The model under review builds one solid part; all positions refer to its coordinate system, in mm. Face numbers are marked on the shaded views. A direction names the side the tool comes from. Give positions to 0.01 mm unless a question says otherwise; leave off trailing zeros. Order: outer loops, then holes, each group sorted by start corner. A loop starts at its lowest first (then second) coordinate and runs counter-clockwise, first axis right, second up.
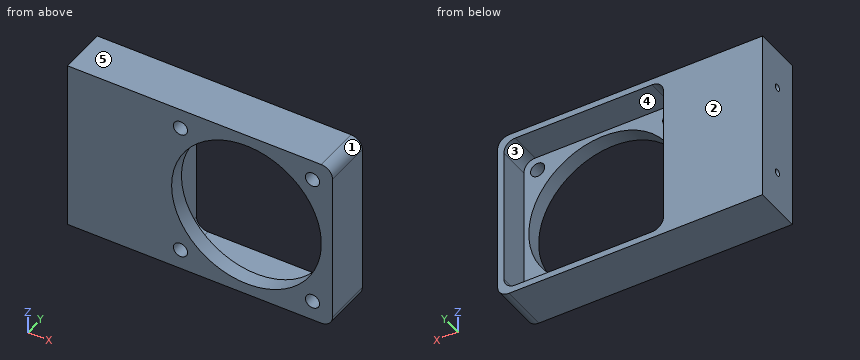
Autodesk Inventor part; units mm, degrees
ref_plane "YZ Plane" through (0, 0, 0) normal (1, 0, 0) x (0, 1, 0)
ref_plane "XZ Plane" through (0, 0, 0) normal (0, 1, 0) x (-1, 0, 0)
ref_plane "XY Plane" through (0, 0, 0) normal (0, 0, 1) x (1, 0, 0)
sketch "Sketch1" plane through (0, 0, 0) normal (0, 1, 0) x (-1, 0, 0)
  line L0 (3.62, 0) -> (84.271, 0)
  line L1 (84.271, 0) -> (84.271, -54.75)
  line L2 (84.271, -54.75) -> (3.62, -54.75)
  line L3 (0, -51.13) -> (0, -3.62)
  circle A0 centre (27.375, -27.375) radius 23.815
  line L4 (0, -27.375) -> (27.375, -27.375) construction
  line L5 (27.375, -27.375) -> (27.375, 0) construction
  arc A1 (0, -51.13) -> (3.62, -54.75) centre (3.62, -51.13) ccw
  arc A2 (3.62, 0) -> (0, -3.62) centre (3.62, -3.62) ccw
  point P0 (0, 0)
  point P1 (0, -54.75)
  dimension "d0" = 54.75
  dimension "d1" = 84.271
  dimension "d2" = 47.63
  dimension "d3" = 3.62
extrude "Extrusion1" add sketch "Sketch1" along normal blind 15.2
sketch "Sketch2" plane through (0, 15.2, 0) normal (0, 1, 0) x (1, 0, 0)
  line L0 (-49.13, 2) -> (-5.62, 2)
  line L1 (-2, 5.62) -> (-2, 49.13)
  line L2 (-5.62, 52.75) -> (-49.13, 52.75)
  line L3 (-52.75, 49.13) -> (-52.75, 5.62)
  circle A0 centre (-27.375, 27.375) radius 23.815 construction
  line L4 (-52.75, 27.375) -> (-2, 27.375) construction
  arc A1 (-52.75, 5.62) -> (-49.13, 2) centre (-49.13, 5.62) ccw
  arc A2 (-49.13, 52.75) -> (-52.75, 49.13) centre (-49.13, 49.13) ccw
  arc A3 (-2, 49.13) -> (-5.62, 52.75) centre (-5.62, 49.13) ccw
  arc A4 (-5.62, 2) -> (-2, 5.62) centre (-5.62, 5.62) ccw
  point P0 (0, 0)
  point P1 (-52.75, 2)
  point P2 (-52.75, 52.75)
  dimension "d6" = 50.75
  dimension "d7" = 3.62
extrude "Extrusion2" cut sketch "Sketch2" against normal blind 10.2
sketch "Sketch3" plane through (0, 5, 0) normal (0, 1, 0) x (1, 0, 0)
  line L0 (-48.375, 6.375) -> (-6.375, 6.375) construction
  line L1 (-6.375, 6.375) -> (-6.375, 48.375) construction
  line L2 (-6.375, 48.375) -> (-48.375, 48.375) construction
  line L3 (-48.375, 48.375) -> (-48.375, 6.375) construction
  line L4 (-48.375, 27.375) -> (-6.375, 27.375) construction
  circle A0 centre (-27.375, 27.375) radius 23.815 construction
  point P0 (0, 0)
  dimension "d10" = 42
hole "Hole1" at (-48.375, 5, -6.375) at (-48.375, 5, -48.375) at (-6.375, 5, -48.375) at (-6.375, 5, -6.375) direction (0, -1, 0) diameter 4.4958 end through all
sketch "Sketch4" plane through (-84.271, 0, -54.75) normal (-1, 0, 0) x (0, 0, 1)
  line L0 (0, 0) -> (54.75, 0) construction
  line L1 (54.75, 0) -> (54.75, 15.2) construction
  line L2 (0, 15.2) -> (54.75, 15.2) construction
  line L3 (0, 0) -> (0, 15.2) construction
  line L4 (12.7, 7.6) -> (42.05, 7.6) construction
  line L5 (51.13, 15.2) -> (3.62, 15.2) construction
  line L6 (27.375, 15.2) -> (27.375, 0) construction
  line L7 (51.19, 0) -> (3.56, 0) construction
  point P0 (27.375, 7.6)
  dimension "d18" = 12.7
  dimension "Bracket_Hole_Spacing" = 29.35
hole "Hole2" at (-84.271, 7.6, -42.05) at (-84.271, 7.6, -12.7) direction (1, 0, 0) diameter 2.159 depth 25.4 tip angle 118
equation "\"d2\" = Fan_ID"
equation "\"d3\" = Fan_Corner_Radius"
equation "\"d7\" = Fan_Corner_Radius"
equation "\"d8\" = Fan_Thickness"
equation "\"d10\" = Fan_Hole_Spacing"
equation "\"Compressor_Center_Offset\" = 56.896"
properties part number "Fan_Bracket" material "ABS Plastic"
Item 1: For the marked faces 4 and 5, list the 3-axis set-ups (+Z, -Z, +X, -X, +Y, -Y) from which the entire face can be reached by the end or side of a thin tool; tool diameter is ignored.
Values found:
face 4: +Y
face 5: +Z, +X, -X, +Y, -Y
Item 2: Take a section at C-C (x = -29.5). Give the boundary of the cut face in (y, z) (3 decimals), and give its area (4 significant figures).
Values found:
outline: (0, -54.75) - (15.2, -54.75) - (15.2, -52.75) - (5, -52.75) - (5, -51.095) - (0, -51.095) - close; (0, -3.655) - (5, -3.655) - (5, -2) - (15.2, -2) - (15.2, 0) - (0, 0) - close
area: 77.35 mm2
Item 3: Take a section at B-B (x = -12). Give the boundary of the cut face in (y, z), and give its area (3 significant figures).
Values found:
outline: (0, -54.75) - (15.2, -54.75) - (15.2, -52.75) - (5, -52.75) - (5, -45.56) - (0, -45.56) - close; (0, -9.19) - (5, -9.19) - (5, -2) - (15.2, -2) - (15.2, 0) - (0, 0) - close
area: 133 mm2
Item 4: Clearance check with flat-ended pins moving along their axes: pin 1 Ø4 at (x, z) = (-6.375, -6.375) entering from -Y; pin 2 Ø3 at (x, z) = (-50.5, -42.5) entering from +Y; pin 3 Ø1.9 at (y, z) = (7.6, -12.7) entering from -X. State where each tip first meets the part, or that it passes through.
Values found:
pin 1: passes through
pin 2: stops at y = 5
pin 3: stops at x = -58.79
Item 5: Take a section at A-A (y = 14). Give the boundary of the cut face in (x, z).
Values found:
outline: (-84.27, -54.75) - (-3.62, -54.75) arc R3.62 ccw to (0, -51.13) - (0, -3.62) arc R3.62 ccw to (-3.62, 0) - (-84.27, 0) - close; hole (-52.75, -49.13) arc R3.62 ccw to (-49.13, -52.75) - (-5.62, -52.75) arc R3.62 ccw to (-2, -49.13) - (-2, -5.62) arc R3.62 ccw to (-5.62, -2) - (-49.13, -2) arc R3.62 ccw to (-52.75, -5.62) - close
Item 6: For line 1 (X direction, y = 14.5, z = -46.5); line 2 (Z direction, x = -80, y = 7); line 3 (Z direction, x = -24, y = 10.25), list the stretches that pass through material, from the lowest coordinate up.
Values found:
line 1: x = -84.27 to -52.75, -2 to 0
line 2: z = -54.75 to -42.95, -41.15 to -13.6, -11.8 to 0
line 3: z = -54.75 to -52.75, -2 to 0
Item 7: Draft analysis for pull direction Z (two halves, no side actions). For the marked faces 1, 2 and 3, state which applies: released by +Z, released by -Z, zero draft, split by the parting line, or undercut.
Values found:
face 1: released by +Z
face 2: zero draft
face 3: undercut
